```python
from build123d import *

# Parameters (mm, degrees)
SKETCH1_R                    = 125
SKETCH1_R_2                  = 4
BOSS_EXTRUDE1_DEPTH          = 6
SKETCH2_R                    = 2.5
BYPASS_HOLE_FOR_SPRING_DEPTH = 177.878489365
SKETCH5_R                    = 45
BYPASS_HOLE_DEPTH            = 10
SKETCH7_R                    = 2.5
CUT_EXTRUDE3_DEPTH           = 177.878489365
SKETCH10_R                   = 7.5
WIRING_PASS_THROUGH_DEPTH    = 6
SKETCH11_W                   = 25
SKETCH11_H                   = 25
CUT_EXTRUDE7_DEPTH           = 10
FILLET2_R                    = 12.5
FILLET3_R                    = 10
SKETCH13_R                   = 2.5
SKETCH13_R_2                 = 3
CUT_EXTRUDE9_DEPTH           = 10
SKETCH14_W                   = 5
SKETCH14_H                   = 25
CUT_EXTRUDE10_DEPTH          = 6


with BuildPart() as part:
    # Sketch1 → Boss-Extrude1 (new body)
    with BuildSketch(Plane(origin=(0, 0, 0), x_dir=(1, 0, 0), z_dir=(0, 1, 0))):
        with Locations(Location((0, 0, 0), (0, 0, 270))):
            Circle(SKETCH1_R)
        with Locations(Location((-96, 0, 0), (0, 0, 270))):
            Circle(SKETCH1_R_2, mode=Mode.SUBTRACT)
        with Locations(Location((-60, 0, 0), (0, 0, 270))):
            Circle(SKETCH1_R_2, mode=Mode.SUBTRACT)
    extrude(amount=BOSS_EXTRUDE1_DEPTH)

    # Sketch2 → Bypass Hole for Spring (cut, through all)
    with BuildSketch(Plane(origin=(0, 0, 0), x_dir=(1, 0, 0), z_dir=(0, 1, 0))):
        with Locations(Location((-77.781745931, 77.781745931, 0), (0, 0, 270))):
            Circle(SKETCH2_R)
        with Locations(Location((77.781745931, 77.781745931, 0), (0, 0, 270))):
            Circle(SKETCH2_R)
        with Locations(Location((77.781745931, -77.781745931, 0), (0, 0, 270))):
            Circle(SKETCH2_R)
        with Locations(Location((-77.781745931, -77.781745931, 0), (0, 0, 270))):
            Circle(SKETCH2_R)
    extrude(amount=BYPASS_HOLE_FOR_SPRING_DEPTH, mode=Mode.SUBTRACT)

    # Sketch5 → Bypass Hole (cut)
    with BuildSketch(Plane(origin=(0, 0, 0), x_dir=(1, 0, 0), z_dir=(0, 1, 0))):
        with Locations(Location((-8, 0, 0), (0, 0, 270))):
            Circle(SKETCH5_R)
    extrude(amount=BYPASS_HOLE_DEPTH, mode=Mode.SUBTRACT)

    # Sketch7 → Cut-Extrude3 (cut, through all)
    with BuildSketch(Plane(origin=(0, 0, 0), x_dir=(1, 0, 0), z_dir=(0, 1, 0))):
        with Locations(Location((100, 29, 0), (0, 0, 270))):
            Circle(SKETCH7_R)
        with Locations(Location((100, -29, 0), (0, 0, 90))):
            Circle(SKETCH7_R)
    extrude(amount=CUT_EXTRUDE3_DEPTH, mode=Mode.SUBTRACT)

    # Sketch10 → Wiring Pass Through (cut)
    with BuildSketch(Plane(origin=(0, 0, 0), x_dir=(1, 0, 0), z_dir=(0, 1, 0))):
        with Locations(Location((77.5, 0, 0), (0, 0, 270))):
            Circle(SKETCH10_R)
    extrude(amount=WIRING_PASS_THROUGH_DEPTH, mode=Mode.SUBTRACT)

    # Sketch11 → Cut-Extrude7 (cut)
    with BuildSketch(Plane(origin=(0, 0, 0), x_dir=(1, 0, 0), z_dir=(0, 1, 0))):
        with Locations((-122.5, 0)):
            Rectangle(SKETCH11_W, SKETCH11_H)
    extrude(amount=CUT_EXTRUDE7_DEPTH, mode=Mode.SUBTRACT)

    # Fillet2
    fillet2_edges = [part.edges().sort_by_distance(p)[0] for p in [
        (-110, 3, 12.5),
        (-110, 3, -12.5),
    ]]
    fillet(fillet2_edges, radius=FILLET2_R - 0.0001)  # a hair under: the kernel refuses the full size

    # Fillet3
    fillet3_edges = [part.edges().sort_by_distance(p)[0] for p in [
        (-124.373429638, 3, 12.5),
        (-124.373429638, 3, -12.5),
    ]]
    fillet(fillet3_edges, radius=FILLET3_R)

    # Sketch13 → Cut-Extrude9 (cut)
    with BuildSketch(Plane(origin=(0, 0, 0), x_dir=(1, 0, 0), z_dir=(0, 1, 0))):
        with Locations(Location((76.013978978, -61.871843354, 0), (0, 0, 270))):
            Circle(SKETCH13_R)
        with Locations(Location((61.871843354, -76.013978977, 0), (0, 0, 270))):
            Circle(SKETCH13_R)
        with Locations(Location((84.499260352, -84.499260352, 0), (0, 0, 270))):
            Circle(SKETCH13_R_2)
        with Locations(Location((-61.871843354, -76.013978978, 0), (0, 0, 270))):
            Circle(SKETCH13_R)
        with Locations(Location((-76.013978977, -61.871843354, 0), (0, 0, 270))):
            Circle(SKETCH13_R)
        with Locations(Location((-84.499260352, -84.499260352, 0), (0, 0, 270))):
            Circle(SKETCH13_R_2)
        with Locations(Location((-76.013978978, 61.871843354, 0), (0, 0, 270))):
            Circle(SKETCH13_R)
        with Locations(Location((-61.871843354, 76.013978977, 0), (0, 0, 270))):
            Circle(SKETCH13_R)
        with Locations(Location((-84.499260352, 84.499260352, 0), (0, 0, 270))):
            Circle(SKETCH13_R_2)
        with Locations(Location((61.871843354, 76.013978978, 0), (0, 0, 270))):
            Circle(SKETCH13_R)
        with Locations(Location((76.013978977, 61.871843354, 0), (0, 0, 270))):
            Circle(SKETCH13_R)
        with Locations(Location((84.499260352, 84.499260352, 0), (0, 0, 270))):
            Circle(SKETCH13_R_2)
    extrude(amount=CUT_EXTRUDE9_DEPTH, mode=Mode.SUBTRACT)

    # Sketch14 → Cut-Extrude10 (cut)
    with BuildSketch(Plane(origin=(0, 0, 0), x_dir=(1, 0, 0), z_dir=(0, 1, 0))):
        with Locations((60, 0)):
            Rectangle(SKETCH14_W, SKETCH14_H)
    extrude(amount=CUT_EXTRUDE10_DEPTH, mode=Mode.SUBTRACT)


solid = part.part
```
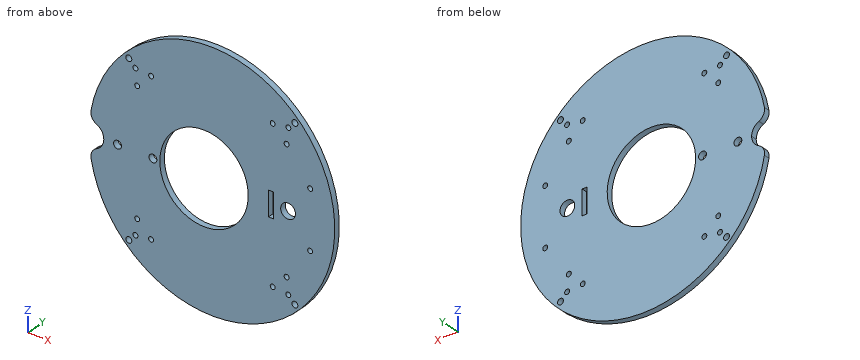
The model under review builds one solid part; all positions refer to its coordinate system, in mm. Round coordinates to 2 decimals unless told otherwise and drop trailing zeros. Write each loop counter-clockwise with the first axis right and the second up, starting at its lowest first coordinate (ties: lowest second). Pieces come first, ordered by that corner, then holes. Notation, with made-up numbers: M 13,17.5 L 26,17.5 A25 ccw 26,45.5 Z; hole C 27,3 d6. An arc over 180 degrees is marked long. Use CSV: the item, a comma, the result in double quotes. Start each with the question number.
(1) We need section D-D, the plane y = 3.5. State how many separate pieces and enclosed holes the cut face has, then the cut area to 3 significant figures.
(2) Clearance check with flat-ended pins moving along their axes: P1, Ø4, axis at x = 61.87, z = -76.01, coming from the +Y side (3 decimals); P2, Ø1, axis at y = 5, z = 8.5, coming from the -X side; P3, Ø3, axis at y = 2, z = 5, coming from the +X side; P4, Ø3, axis at x = 70.5, y = 0.5, coming from the +Z side. State where each tip first meets the part, or that it passes through.
(3) We need section B-B, the plane x = -96. State the section outline as (y, z) points.
(4) We need section A-A, the plane x = 12.5. State the section outline as (y, z) points.
(5) For line 1 along Z through (x, y) = (64, 3.5); line 2 along Z through (x, y) = (-84, 2.75); line 3 along Z through (x, y) = (-61, 5.5), list the stretches that pass through material, from the lowest coordinate up.
(6) We need section C-C, the plane z = -102. State the section outline as (x, y) points.
Findings:
1,separate pieces,"1"
1,enclosed holes,"23"
1,area,"41,600 mm^2"
2,P1,"through"
2,P2,"x = -113.83"
2,P3,"x = 124.95"
2,P4,"z = 104.23"
3,outline,"M 0,-80.06 L 6,-80.06 L 6,-4 L 0,-4 Z; M 0,4 L 6,4 L 6,80.06 L 0,80.06 Z"
4,outline,"M 0,-124.37 L 6,-124.37 L 6,-40.06 L 0,-40.06 Z; M 0,40.06 L 6,40.06 L 6,124.37 L 0,124.37 Z"
5,line 1,"-107.37 to -77.33, -74.7 to 74.7, 77.33 to 107.37"
5,line 2,"-92.57 to -87.46, -81.54 to 81.54, 87.46 to 92.57"
5,line 3,"-109.11 to -78.36, -73.67 to -3.87, 3.87 to 73.67, 78.36 to 109.11"
6,outline,"M -72.26,0 L 72.26,0 L 72.26,6 L -72.26,6 Z"
